Work out the finished part from the listing and answer in its coordinate system (mm). A direction names the side the tool comes from. Round coordinates to 2 decimals unless told otherwise and drop trailing zeros. Order: outer loops, then holes, each group sorted by start corner. A loop starts at its lowest first (then second) coordinate and runs counter-clockwise, first axis right, second up. Notation, with made-up numbers: (-3, 35) - (19, 35) arc R9 cw to (19, 40) - close; hole circle Ø11 at (7.25, 52.25). An arc over 180 degrees is marked (long way). Use CSV: the item, a comma, the result in double quotes.
from build123d import *

# Parameters (mm, degrees)
F0_W     = 110
F0_H     = 110
F1_DEPTH = 50
F2_W     = 105
F2_H     = 105
F3_DEPTH = 35
F4_W     = 104
F4_H     = 5
F5_DEPTH = 108
F6_W     = 12.735002
F6_H     = 6.483276
F6_W_2   = 7.409461
F6_H_2   = 6.483274
F7_DEPTH = 50
F8_R     = 2.5


with BuildPart() as f1:
    # F0 (on Top) → F1 (new body)
    with BuildSketch(Plane.XY):
        Rectangle(F0_W, F0_H)
    extrude(amount=F1_DEPTH)

    # F2 (on face) → F3 (cut)
    with BuildSketch(Plane.XY.offset(50)):
        Rectangle(F2_W, F2_H)
    extrude(amount=-F3_DEPTH, mode=Mode.SUBTRACT)

    # F4 (on face) → F5 (cut)
    with BuildSketch(Plane(origin=(0, 55, 0), x_dir=(-1, 0, 0), z_dir=(0, 1, 0))):
        with Locations((0, 46.881082)):
            Rectangle(F4_W, F4_H)
    extrude(amount=-F5_DEPTH, mode=Mode.SUBTRACT)

    # F6 (on face) → F7 (cut)
    with BuildSketch(Plane(origin=(0, 55, 0), x_dir=(-1, 0, 0), z_dir=(0, 1, 0))):
        with Locations((-41.632924, 35.490146)):
            Rectangle(F6_W, F6_H)
        with Locations((43.460033, 10.946326)):
            Rectangle(F6_W_2, F6_H_2)
    extrude(amount=-F7_DEPTH, mode=Mode.SUBTRACT)

    # F8
    f8_edges = [f1.edges().sort_by_distance(p)[0] for p in [
        (-55, 55, 25),
        (-55, -55, 25),
        (55, 55, 25),
        (55, -55, 25),
    ]]
    fillet(f8_edges, radius=F8_R)


solid = f1.part
(1) For faces 4 (the flat face through (-52.5, -1, 33)), 5 (the flat face through (42, 54, 38.732)), 6 (the cylindrical face through (-54.287, 54.248, 25.35)), determine the directions among +Z, -Z, +X, -X, +Y, -Y from which every point of the face is accessible in a straight line to the end or side of a thin tool.
Findings below:
face 4,"+Z"
face 5,"+Y"
face 6,"+Z, -Z, -X, +Y"
(2) Find section C-C (z = 21.5). Determine the outline of the cut face in (x, y), and give its area (3 significant figures).
Findings below:
outline,"(-55, -52.5) arc R2.5 ccw to (-52.5, -55) - (52.5, -55) arc R2.5 ccw to (55, -52.5) - (55, 52.5) arc R2.5 ccw to (52.5, 55) - (-52.5, 55) arc R2.5 ccw to (-55, 52.5) - close; hole (-52.5, -52.5) - (52.5, -52.5) - (52.5, 52.5) - (-52.5, 52.5) - close"
area,"1,070 mm²"
(3) Find section A-A (x = 18). Determine the outline of the cut face in (y, z), and give its area (3 significant figures).
Findings below:
outline,"(-55, 0) - (55, 0) - (55, 44.38) - (52.5, 44.38) - (52.5, 15) - (-52.5, 15) - (-52.5, 44.38) - (-53, 44.38) - (-53, 49.38) - (-52.5, 49.38) - (-52.5, 50) - (-55, 50) - close; (52.5, 49.38) - (55, 49.38) - (55, 50) - (52.5, 50) - close"
area,"1,810 mm²"
(4) Find section D-D (x = 43.5). Determine the outline of the cut face in (y, z).
Findings below:
outline,"(-55, 0) - (55, 0) - (55, 32.25) - (52.5, 32.25) - (52.5, 15) - (-52.5, 15) - (-52.5, 44.38) - (-53, 44.38) - (-53, 49.38) - (-52.5, 49.38) - (-52.5, 50) - (-55, 50) - close; (52.5, 38.73) - (55, 38.73) - (55, 44.38) - (52.5, 44.38) - close; (52.5, 49.38) - (55, 49.38) - (55, 50) - (52.5, 50) - close"
(5) The mould has two halves that part along Z. Classify faces 1 (the flat face through (-1, 52.5, 29)), 2 (the flat face through (-4, -53, 50)), 3 (the flat face through (1, 54, 49.381)): released by +Z, released by -Z, zero draft, split by the parting line, or undercut.
Findings below:
face 1,"zero draft"
face 2,"released by +Z"
face 3,"undercut"
(6) Each of these flat-tipped pins is pushed along its axis until it touches: pin 1 (2 mm diameter, centred on x = 21.5, y = 24, fed in from +Z); pin 2 (0.6 mm diameter, centred on y = -53, z = 46, fed in from -X); pin 3 (0.8 mm diameter, centred on y = 53.5, z = 46, fed in from +X). Where does it stop, or does it pass through?
Findings below:
pin 1,"stops at z = 15"
pin 2,"stops at x = -54.99"
pin 3,"stops at x = 54.93"
(7) Find section B-B (y = 34). Determine the outline of the cut face in (x, z), and give its area (3 significant figures).
Findings below:
outline,"(-55, 0) - (55, 0) - (55, 50) - (52.5, 50) - (52.5, 15) - (-52.5, 15) - (-52.5, 50) - (-55, 50) - close; hole (-47.16, 7.7) - (-39.76, 7.7) - (-39.76, 14.19) - (-47.16, 14.19) - close"
area,"1,780 mm²"
(8) Find the intervals of material crossed by L1, parallel to X at y = 50.5, z = 29.5; L2, parallel to Z at x = -46.5, y = 38.5, in increasing order. Write a range as from..to.
Findings below:
L1,"x = -55..-52.5, 52.5..55"
L2,"z = 0..7.7, 14.19..15"
